Check sheet for the modelled part. Datum: model origin and axes. Units: mm. Face numbers are marked on the shaded views. A direction names the side the tool comes from. Coordinates: 2 decimals unless noted, no trailing zeros. Loops run counter-clockwise (first coordinate to the right, second up) from the corner with the lowest first, then second, coordinate; pieces in that order, holes last.
from build123d import *

# Parameters (mm, degrees)
BOSS_EXTRU_1_DEPTH      = 4
ESQUISSE2_R             = 1.5
ENL_V_MAT_EXTRU_1_DEPTH = 4
ESQUISSE3_W             = 5
ESQUISSE3_H             = 4
BOSS_EXTRU_2_DEPTH      = 12
BOSS_EXTRU_3_DEPTH      = 4
ESQUISSE5_R             = 1.5
ENL_V_MAT_EXTRU_2_DEPTH = 4
CHANFREIN2_SIZE         = 2
ESQUISSE6_W             = 20
ESQUISSE6_H             = 5
BOSS_EXTRU_4_DEPTH      = 10
CONG_1_R                = 5
ESQUISSE7_R             = 1.5
ENL_V_MAT_EXTRU_3_DEPTH = 10


with BuildPart() as part:
    # Esquisse1 → Boss.-Extru.1 (new body)
    with BuildSketch(Plane.XY):
        with BuildLine():
            Line((0, 0), (0, -53))
            ThreePointArc((0, -53), (1.464466094, -56.535533906), (5, -58))
            Line((5, -58), (55, -58))
            ThreePointArc((55, -58), (58.535533906, -56.535533906), (60, -53))
            Line((60, -53), (60, 0))
            Line((60, 0), (0, 0))
        make_face()
    extrude(amount=BOSS_EXTRU_1_DEPTH)

    # Esquisse2 → Enlèv. mat.-Extru.1 (cut)
    with BuildSketch(Plane.XY.offset(4)):
        with Locations((13.397040157, -7.66880337)):
            Circle(ESQUISSE2_R)
        with Locations((4.459764877, -53.98621161)):
            Circle(ESQUISSE2_R)
        with Locations((55.540235123, -53.98621161)):
            Circle(ESQUISSE2_R)
        with Locations((46.602959843, -7.66880337)):
            Circle(ESQUISSE2_R)
    extrude(amount=-ENL_V_MAT_EXTRU_1_DEPTH, mode=Mode.SUBTRACT)

    # Esquisse3 → Boss.-Extru.2 (add)
    with BuildSketch(Plane(origin=(0, 0, 0), x_dir=(-1, 0, 0), z_dir=(0, 0, -1))):
        with Locations((-38.5, -2)):
            Rectangle(ESQUISSE3_W, ESQUISSE3_H)
        with Locations((-10.5, -2)):
            Rectangle(ESQUISSE3_W, ESQUISSE3_H)
    extrude(amount=BOSS_EXTRU_2_DEPTH)

    # Esquisse4 → Boss.-Extru.3 (add)
    with BuildSketch(Plane(origin=(0, 0, 0), x_dir=(1, 0, 0), z_dir=(0, 1, 0))):
        with BuildLine():
            Line((0, 0), (8, 0))
            Line((8, 0), (8, 12))
            Line((8, 12), (5, 12))
            ThreePointArc((5, 12), (1.464466094, 10.535533906), (0, 7))
            Line((0, 7), (0, 0))
        make_face()
        with BuildLine():
            Line((60, 0), (41, 0))
            Line((41, 0), (41, 12))
            Line((41, 12), (55, 12))
            ThreePointArc((55, 12), (58.535533906, 10.535533906), (60, 7))
            Line((60, 7), (60, 0))
        make_face()
    extrude(amount=-BOSS_EXTRU_3_DEPTH)

    # Esquisse5 → Enlèv. mat.-Extru.2 (cut)
    with BuildSketch(Plane(origin=(0, 0, 0), x_dir=(1, 0, 0), z_dir=(0, 1, 0))):
        with Locations((10.5, 6)):
            Circle(ESQUISSE5_R)
        with Locations((38.5, 6)):
            Circle(ESQUISSE5_R)
    extrude(amount=-ENL_V_MAT_EXTRU_2_DEPTH, mode=Mode.SUBTRACT)

    # Chanfrein2
    chanfrein2_edges = [part.edges().sort_by_distance(p)[0] for p in [
        (45.102959843, -7.66880337, 0),
        (11.897040157, -7.66880337, 0),
    ]]
    chamfer(chanfrein2_edges, length=CHANFREIN2_SIZE)

    # Esquisse6 → Boss.-Extru.4 (add)
    with BuildSketch(Plane(origin=(0, 0, 0), x_dir=(-1, 0, 0), z_dir=(0, 0, -1))):
        with Locations((-29.497744904, -55.5)):
            Rectangle(ESQUISSE6_W, ESQUISSE6_H)
    extrude(amount=BOSS_EXTRU_4_DEPTH)

    # Congé1
    cong_1_edges = [part.edges().sort_by_distance(p)[0] for p in [
        (39.497744904, -55.5, -10),
        (19.497744904, -55.5, -10),
    ]]
    fillet(cong_1_edges, radius=CONG_1_R)

    # Esquisse7 → Enlèv. mat.-Extru.3 (cut)
    with BuildSketch(Plane.XZ.offset(58)):
        with Locations((29.497744904, -5)):
            Circle(ESQUISSE7_R)
    extrude(amount=-ENL_V_MAT_EXTRU_3_DEPTH, mode=Mode.SUBTRACT)


solid = part.part
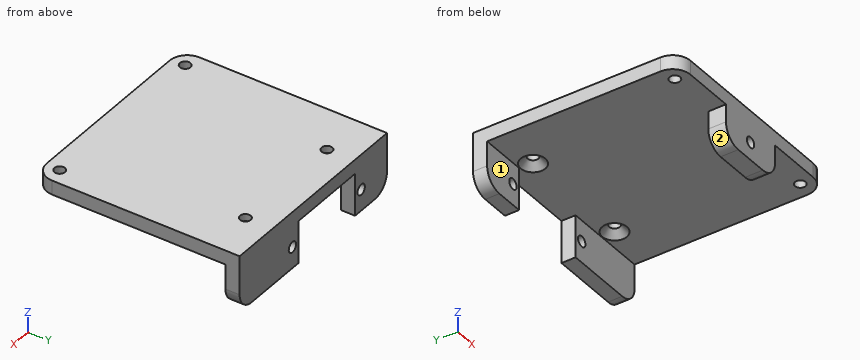
(1) Section check B-B, the plane x = 38.5. Enter the section's corners in (y, z).
(2) Section check C-C, the plane y = -37. Enter the section's corners in (x, z).
(3) Gauge pin test, flat ends, axial feed: P1, Ø8, axis at x = 52.5, y = -45, coming from the -Z side; P2, Ø3.5, axis at x = 10.5, z = -6, coming from the -Y side; P3, Ø2.5, axis at x = 38.5, z = -6, coming from the +Y side; P4, Ø1.8, axis at x = 13.4, y = -7.67, coming from the +Z side. Record the tip position at first contact, or that the pin passes through.
(4) Section check D-D, the plane x = 18. Enter the section's corners in (y, z), plus the area to 3 significant figures.
(5) Scan lines: line 1 along X through (y, z) = (-1.5, -6); line 2 along Z through (x, y) = (38.5, -0.85); line 3 along X through (y, z) = (-8, 0.5). Record each from-to range of solid material in increasing order.
(6) Set-up check for the marked faces 1 and 2: record each of +Z, -Z, +X, -X, +Y, -Y from which the full face is reachable in a straight line by a thin tool's end or side.
(7) Section check A-A, the plane x = 29.5. Enter the section's corners in (y, z), plus the area to 3 significant figures.
Determined:
1. outline: (-58, -8) - (-53, -8) - (-53, 0) - (-4, 0) - (-4, -4.5) - (0, -4.5) - (0, 4) - (-58, 4) - close; (-4, -12) - (0, -12) - (0, -7.5) - (-4, -7.5) - close
2. outline: (0, 0) - (60, 0) - (60, 4) - (0, 4) - close
3. P1: stops at z = 0
3. P2: stops at y = -4
3. P3: stops at y = -53
3. P4: passes through
4. outline: (-58, 0) - (0, 0) - (0, 4) - (-58, 4) - close
4. area: 232 mm2
5. line 1: x = 0 to 9, 12 to 13, 36 to 37, 40 to 60
5. line 2: z = -12 to -7.5, -4.5 to 4
5. line 3: x = 0 to 10.42, 16.38 to 43.62, 49.58 to 60
6. face 1: -Z, +X, -X, -Y
6. face 2: -Z, -X, +Y, -Y
7. outline: (-58, -10) - (-53, -10) - (-53, -6.5) - (-58, -6.5) - close; (-58, -3.5) - (-53, -3.5) - (-53, 0) - (0, 0) - (0, 4) - (-58, 4) - close
7. area: 267 mm2
